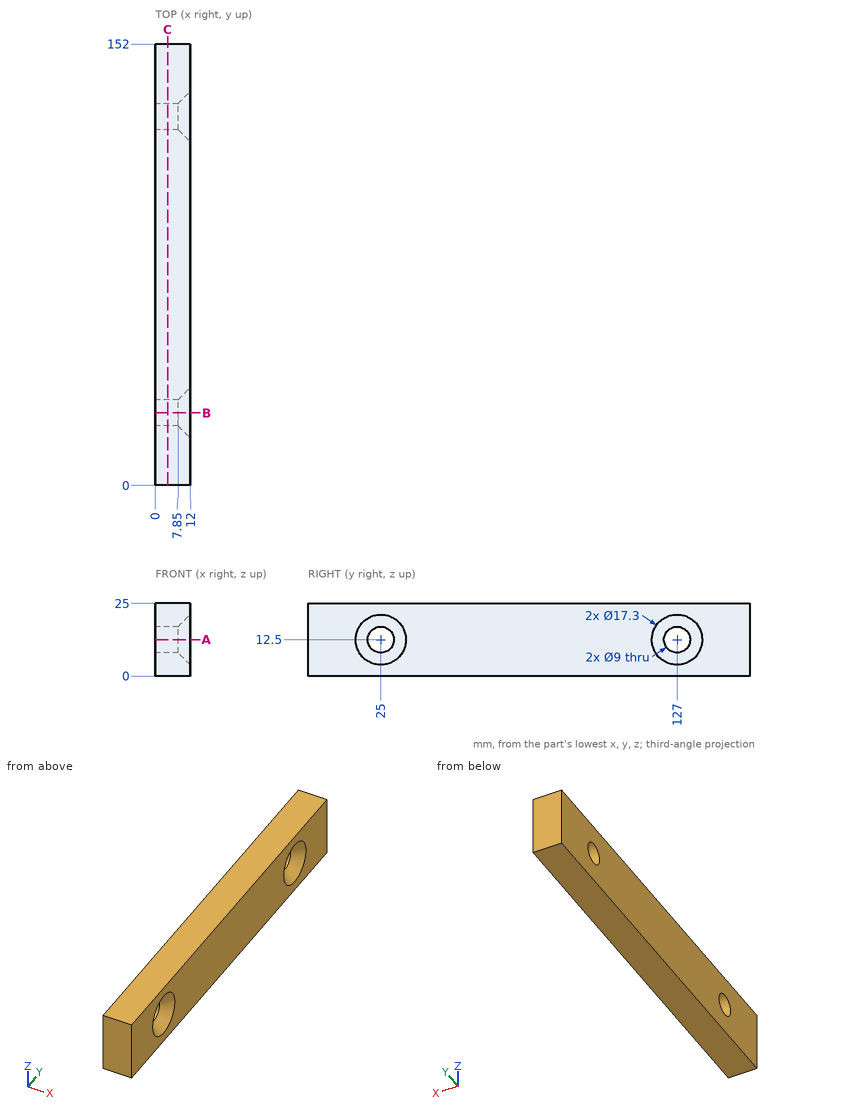
The drawing under review shows one solid part. Ordinate dimensions are in mm from its lowest x, y, z. Give positions to 0.01 mm unless a question says otherwise; leave off trailing zeros. Write each loop counter-clockwise with the first axis right and the second up, starting at its lowest first coordinate (ties: lowest second). Pieces come first, ordered by that corner, then holes.
1. For P1, Ø14.5, axis at y = 127, z = 12.5, coming from the +X side, flat-tipped, find the tip position at first contact; note if it passes through.
2. Add section A-A, the plane z = 12.5. Write out the cut boundary in (x, y).
3. Wall thickness on L1, parallel to Y at x = 3.25, z = 13; L2, parallel to Z at x = 5.75, y = 127; L3, parallel to Y at x = 0.5, z = 11.5: over which ranges is each line inside the solid? List them lowest first.
4. Add section B-B, the plane y = 25. Write out the cut boundary in (x, z).
5. Add section C-C, the plane x = 4.25. Write out the cut boundary in (y, z), plus the area to 3 significant figures.
Worked answers:
1. P1: stops at x = 10.6
2. outline: (0, 0) - (12, 0) - (12, 16.35) - (7.85, 20.5) - (0, 20.5) - close; (0, 29.5) - (7.85, 29.5) - (12, 33.65) - (12, 118.35) - (7.85, 122.5) - (0, 122.5) - close; (0, 131.5) - (7.85, 131.5) - (12, 135.65) - (12, 152) - (0, 152) - close
3. L1: y = 0 to 20.53, 29.47 to 122.53, 131.47 to 152
3. L2: z = 0 to 8, 17 to 25
3. L3: y = 0 to 20.61, 29.39 to 122.61, 131.39 to 152
4. outline: (0, 0) - (12, 0) - (12, 3.85) - (7.85, 8) - (0, 8) - close; (0, 17) - (7.85, 17) - (12, 21.15) - (12, 25) - (0, 25) - close
5. outline: (0, 0) - (152, 0) - (152, 25) - (0, 25) - close; hole circle Ø9 at (25, 12.5); hole circle Ø9 at (127, 12.5)
5. area: 3,670 mm2
